```python
from build123d import *

# Parameters (mm, degrees)
F0_W      = 4.572
F0_H      = 45.466
F0_H_2    = 31.242
F0_H_3    = 35.814
F0_H_4    = 37.846
F0_H_5    = 36.83
F0_H_6    = 37.338
F0_H_7    = 36.322
F1_DEPTH  = 10.922
F3_DEPTH  = 10.923
F5_DEPTH  = 10.923
F6_W      = 4.572
F6_H      = 45.466
F7_DEPTH  = 4.826
F8_W      = 4.572
F8_H      = 35.814
F9_DEPTH  = 4.826
F10_W     = 4.572
F10_H     = 36.83
F11_DEPTH = 4.826
F12_W     = 4.572
F12_H     = 35.814
F13_DEPTH = 4.826
F14_W     = 4.572
F14_H     = 37.338
F15_DEPTH = 4.826
F16_W     = 4.572
F16_H     = 36.322
F17_DEPTH = 4.826
F18_W     = 4.572
F18_H     = 37.338
F19_DEPTH = 4.826
F20_W     = 4.572
F20_H     = 37.846
F21_DEPTH = 4.826
F22_W     = 4.572
F22_H     = 31.242
F23_DEPTH = 4.826
F24_W     = 38.862
F24_H     = 4.572
F25_DEPTH = 4.826
F26_W     = 38.862
F26_H     = 4.572
F27_DEPTH = 4.826


with BuildPart() as f1:
    # F0 (on Top) → F1 (new body)
    with BuildSketch(Plane.XY):
        with BuildLine():
            Line((-50.638884, 267.268687), (-151.155582, 267.268687))
            ThreePointArc((-151.155582, 267.268687), (-158.160182, 264.367287), (-161.061582, 257.362687))
            Line((-161.061582, 257.362687), (-161.061582, -261.813313))
            ThreePointArc((-161.061582, -261.813313), (-158.160182, -268.817912), (-151.155582, -271.719313))
            Line((-151.155582, -271.719313), (152.882418, -271.719313))
            ThreePointArc((152.882418, -271.719313), (159.887018, -268.817912), (162.788418, -261.813313))
            Line((162.788418, -261.813313), (162.788418, -254.955313))
            Line((162.788418, -254.955313), (158.216418, -254.955313))
            Line((158.216418, -254.955313), (158.216418, -209.489313))
            Line((158.216418, -209.489313), (162.788418, -209.489313))
            Line((162.788418, -209.489313), (162.788418, -188.407313))
            Line((162.788418, -188.407313), (158.216418, -188.407313))
            Line((158.216418, -188.407313), (158.216418, -152.593313))
            Line((158.216418, -152.593313), (162.788418, -152.593313))
            Line((162.788418, -152.593313), (162.788418, -129.733313))
            Line((162.788418, -129.733313), (158.216418, -129.733313))
            Line((158.216418, -129.733313), (158.216418, -92.903313))
            Line((158.216418, -92.903313), (162.788418, -92.903313))
            Line((162.788418, -92.903313), (162.788418, -74.107313))
            Line((162.788418, -74.107313), (158.216418, -74.107313))
            Line((158.216418, -74.107313), (158.216418, -38.293313))
            Line((158.216418, -38.293313), (162.788418, -38.293313))
            Line((162.788418, -38.293313), (162.788418, -15.179313))
            Line((162.788418, -15.179313), (158.216418, -15.179313))
            Line((158.216418, -15.179313), (158.216418, 22.158687))
            Line((158.216418, 22.158687), (162.788418, 22.158687))
            Line((162.788418, 22.158687), (162.788418, 44.764687))
            Line((162.788418, 44.764687), (158.216418, 44.764687))
            Line((158.216418, 44.764687), (158.216418, 81.086687))
            Line((158.216418, 81.086687), (162.788418, 81.086687))
            Line((162.788418, 81.086687), (162.788418, 103.946687))
            Line((162.788418, 103.946687), (158.216418, 103.946687))
            Line((158.216418, 103.946687), (158.216418, 141.284687))
            Line((158.216418, 141.284687), (162.788418, 141.284687))
            Line((162.788418, 141.284687), (162.788418, 162.366687))
            Line((162.788418, 162.366687), (158.216418, 162.366687))
            Line((158.216418, 162.366687), (158.216418, 200.212687))
            Line((158.216418, 200.212687), (162.788418, 200.212687))
            Line((162.788418, 200.212687), (162.788418, 226.120687))
            Line((162.788418, 226.120687), (158.216418, 226.120687))
            Line((158.216418, 226.120687), (158.216418, 257.362687))
            Line((158.216418, 257.362687), (162.788418, 257.362687))
            ThreePointArc((162.788418, 257.362687), (159.887018, 264.367287), (152.882418, 267.268687))
            Line((152.882418, 267.268687), (66.598618, 267.268687))
            Line((66.598618, 267.268687), (56.692618, 267.268687))
            Line((56.692618, 267.268687), (56.03563, 267.268687))
            Line((56.03563, 267.268687), (-40.811159, 267.268687))
            Line((-40.811159, 267.268687), (-41.249528, 267.268687))
            Line((-41.249528, 267.268687), (-50.638884, 267.268687))
        make_face()
        with Locations((160.502418, -232.222313)):
            Rectangle(F0_W, F0_H)
        with Locations((160.502418, 241.741687)):
            Rectangle(F0_W, F0_H_2)
        with Locations((160.502418, -170.500313)):
            Rectangle(F0_W, F0_H_3)
        with Locations((160.502418, 181.289687)):
            Rectangle(F0_W, F0_H_4)
        with Locations((160.502418, -111.318313)):
            Rectangle(F0_W, F0_H_5)
        with Locations((160.502418, 122.615687)):
            Rectangle(F0_W, F0_H_6)
        with Locations((160.502418, -56.200313)):
            Rectangle(F0_W, F0_H_3)
        with Locations((160.502418, 62.925687)):
            Rectangle(F0_W, F0_H_7)
        with Locations((160.502418, 3.489687)):
            Rectangle(F0_W, F0_H_6)
    extrude(amount=F1_DEPTH)

    # F2 (on face) → F3 (cut, through all)
    with BuildSketch(Plane.XY.offset(10.922)):
        with BuildLine():
            Line((66.59181, 267.268687), (-50.65459, 267.268687))
            ThreePointArc((-50.65459, 267.268687), (-47.75319, 260.264088), (-40.74859, 257.362687))
            Line((-40.74859, 257.362687), (56.68581, 257.362687))
            ThreePointArc((56.68581, 257.362687), (63.69041, 260.264088), (66.59181, 267.268687))
        make_face()
    extrude(amount=-F3_DEPTH, mode=Mode.SUBTRACT)

    # F4 (on face) → F5 (cut, through all)
    with BuildSketch(Plane.XY.offset(10.922)):
        with BuildLine():
            Line((56.699284, -261.813313), (-40.735632, -261.813313))
            ThreePointArc((-40.735632, -261.813313), (-47.740232, -264.714713), (-50.641632, -271.719313))
            Line((-50.641632, -271.719313), (-50.641632, -271.741477))
            Line((-50.641632, -271.741477), (66.605284, -271.741477))
            Line((66.605284, -271.741477), (66.605284, -271.719313))
            ThreePointArc((66.605284, -271.719313), (63.703884, -264.714713), (56.699284, -261.813313))
        make_face()
    extrude(amount=-F5_DEPTH, mode=Mode.SUBTRACT)

    # F6 (on face) → F7 (join)
    with BuildSketch(Plane.XY.offset(10.922)):
        with Locations((160.516776, -232.222313)):
            Rectangle(F6_W, F6_H)
    extrude(amount=F7_DEPTH)

    # F8 (on face) → F9 (join)
    with BuildSketch(Plane.XY.offset(10.922)):
        with Locations((160.412975, -170.500313)):
            Rectangle(F8_W, F8_H)
    extrude(amount=F9_DEPTH)

    # F10 (on face) → F11 (join)
    with BuildSketch(Plane.XY.offset(10.922)):
        with Locations((160.571285, -111.318313)):
            Rectangle(F10_W, F10_H)
    extrude(amount=F11_DEPTH)

    # F12 (on face) → F13 (join)
    with BuildSketch(Plane.XY.offset(10.922)):
        with Locations((160.571292, -56.200313)):
            Rectangle(F12_W, F12_H)
    extrude(amount=F13_DEPTH)

    # F14 (on face) → F15 (join)
    with BuildSketch(Plane.XY.offset(10.922)):
        with Locations((160.397649, 3.489687)):
            Rectangle(F14_W, F14_H)
    extrude(amount=F15_DEPTH)

    # F16 (on face) → F17 (join)
    with BuildSketch(Plane.XY.offset(10.922)):
        with Locations((160.66844, 62.925687)):
            Rectangle(F16_W, F16_H)
    extrude(amount=F17_DEPTH)

    # F18 (on face) → F19 (join)
    with BuildSketch(Plane.XY.offset(10.922)):
        with Locations((160.713606, 122.615687)):
            Rectangle(F18_W, F18_H)
    extrude(amount=F19_DEPTH)

    # F20 (on face) → F21 (join)
    with BuildSketch(Plane.XY.offset(10.922)):
        with Locations((160.567634, 181.289687)):
            Rectangle(F20_W, F20_H)
    extrude(amount=F21_DEPTH)

    # F22 (on face) → F23 (join)
    with BuildSketch(Plane.XY.offset(10.922)):
        with Locations((160.567634, 241.741687)):
            Rectangle(F22_W, F22_H)
    extrude(amount=F23_DEPTH)

    # F24 (on face) → F25 (join)
    with BuildSketch(Plane.XY.offset(10.922)):
        with Locations((108.051418, 264.982687)):
            Rectangle(F24_W, F24_H)
    extrude(amount=F25_DEPTH)

    # F26 (on face) → F27 (join)
    with BuildSketch(Plane.XY.offset(10.922)):
        with Locations((108.051418, -269.433313)):
            Rectangle(F26_W, F26_H)
    extrude(amount=F27_DEPTH)


solid = f1.part
```
Source: CAD feature listing. Evaluate the final solid. Frame: model axes, mm. A direction names the side the tool comes from. Coordinates: 2 decimals unless noted, no trailing zeros. Write each loop counter-clockwise with the first axis right and the second up, starting at its lowest first coordinate (ties: lowest second). Pieces come first, ordered by that corner, then holes. Notation, with made-up numbers: (59, -23.5) -> (102, -23.5) arc R26 cw to (102, -5.5) -> close; hole circle Ø7 at (57.25, 43). An arc over 180 degrees is marked (long way). Return JSON: item names as keys, results as strings. Group by question number.
1) Section query B-B, the plane x = 98. Return loops of the section in (y, z), plus the area to 3 significant figures.
2) Mould query, pull axis X, two halves, no side actions, for faces 4 (the face through (159.81, -268.895, 5.385)), 5 (the face through (7, 257.363, 6)), 6 (the face through (109, -271.719, 6)). Classes: +X half, -X half, draft (parallel to the pull), parting line (faces both ways), or undercut.
3) Section query C-C, the plane x = -100. Return loops of the section in (y, z), plus the area to 3 significant figures.
4) Section query D-D, the plane y = -137.5. Return loops of the section in (x, z).
5) Set-up query: faces 1 (the face through (9, -261.813, 6)), 2 (the face through (63.613, 260.187, 5.537)), 3 (the face through (110, 267.269, 6)). Return all of +Z, -Z, +X, -X, +Y, -Y with unobstructed straight access to the full face (end or side cutting, diameter ignored); none if empty.
6) Ray query, line 1 along X through (y, z) = (206.5, 4.75); line 2 along X through (y, z) = (189.5, 11.5); line 3 along Y through (x, z) = (5.5, 2.25). Return the intervals inside material, ascending.
7) Contact query for flat-ended pins moving along their axis: P1, Ø4, axis at y = -172, z = 13.5, coming from the -X side; P2, Ø1.4, axis at y = 244, z = 13, coming from the -X side; P3, Ø2.5, axis at x = 160.5, z = 12.5, coming from the +Y side. Output: stop coordinate, or through.
8) Section query A-A, the plane y = 180.5. Return loops of the section in (x, z).
From the geometry:
{
 "1": {"outline": "(-271.72, 0) -> (267.27, 0) -> (267.27, 15.75) -> (262.7, 15.75) -> (262.7, 10.92) -> (-267.15, 10.92) -> (-267.15, 15.75) -> (-271.72, 15.75) -> close", "area": "5,930 mm²"},
 "2": {"face 4": "+X half", "face 5": "undercut", "face 6": "draft"},
 "3": {"outline": "(-271.72, 0) -> (267.27, 0) -> (267.27, 10.92) -> (-271.72, 10.92) -> close", "area": "5,890 mm²"},
 "4": {"outline": "(-161.06, 0) -> (162.79, 0) -> (162.79, 10.92) -> (-161.06, 10.92) -> close"},
 "5": {"face 1": "+Z, -Z, -Y", "face 2": "+Z, -Z, +Y", "face 3": "+Z, -Z, +X, -X, +Y"},
 "6": {"line 1": "-161.06 to 162.79", "line 2": "158.28 to 162.85", "line 3": "-261.81 to 257.36"},
 "7": {"P1": "x = 158.13", "P2": "x = 158.28", "P3": "y = 257.36"},
 "8": {"outline": "(-161.06, 0) -> (162.79, 0) -> (162.79, 10.92) -> (162.85, 10.92) -> (162.85, 15.75) -> (158.28, 15.75) -> (158.28, 10.92) -> (-161.06, 10.92) -> close"}
}
